Check sheet for the modelled part. Datum: model origin and axes. Units: mm. A direction names the side the tool comes from. Round coordinates to 2 decimals unless told otherwise and drop trailing zeros. Write each loop counter-clockwise with the first axis right and the second up, starting at its lowest first coordinate (ties: lowest second). Pieces come first, ordered by that corner, then holes.
Item 1: Section check C-C, the plane x = 7.75. Record the cut outline in (y, z).
Item 2: Material ranges on line 1 along X through (y, z) = (3.25, 0.8); line 2 along Y through (x, z) = (6.5, 0.45); line 3 along X through (y, z) = (3, 0.8), recorded low to high.
Item 3: Set-up check for faces 1 (the flat face through (0, 7.5, 0.5)), 2 (the cylindrical face through (4.977, -0.483, 0.493)), 3 (the cylindrical face through (-4.413, 2.351, 0.493)), 4 (the flat face through (-1.47, -7.39, 0.49)): record each of +Z, -Z, +X, -X, +Y, -Y from which the full face is reachable in a straight line by a thin tool's end or side.
Item 4: Section check B-B, the plane y = 6. Record the cut outline in (x, z), plus the area to 3 significant figures.
Item 5: Release check for a two-part mould opening along Y. For faces 5 (the flat face through (7.702, -6.303, 0.493)), 6 (the flat face through (-1, 9.9, 0.5)), 7 (the flat face through (-7, 2.9, 0.5)) record: pulls with the +Y half, pulls with the -Y half, needs draft (parallel to the pull), parting line crosses it, or undercut.
Item 6: Section check A-A, the plane x = -3.25. Record the cut outline in (y, z).
Item 7: Depth check by flat-ended pin: pin 1 (2 mm diameter, centred on x = 4.5, y = -4.5, fed in from -Z). Enter the tip coordinate at first touch or a pass-through.
Autodesk Inventor part; units mm, degrees
ref_plane "YZ Plane" through (0, 0, 0) normal (1, 0, 0) x (0, 1, 0)
ref_plane "XZ Plane" through (0, 0, 0) normal (0, 1, 0) x (-1, 0, 0)
ref_plane "XY Plane" through (0, 0, 0) normal (0, 0, 1) x (1, 0, 0)
sketch "Sketch1" plane through (0, 0, 0) normal (0, 0, 1) x (1, 0, 0)
  circle A0 centre (0, 0) radius 1
  circle A1 centre (0, 0) radius 5
  line L0 (1.9509, 9.8079) -> (3.8268, 9.2388)
  line L1 (5.5557, 8.3147) -> (7.0711, 7.0711)
  line L2 (8.3147, 5.5557) -> (9.2388, 3.8268)
  line L3 (9.8079, 1.9509) -> (10, 0)
  line L4 (9.8079, -1.9509) -> (9.2388, -3.8268)
  line L5 (8.3147, -5.5557) -> (7.0711, -7.0711)
  line L6 (5.5557, -8.3147) -> (3.8268, -9.2388)
  line L7 (1.9509, -9.8079) -> (0, -10)
  line L8 (-1.9509, -9.8079) -> (-3.8268, -9.2388)
  line L9 (-5.5557, -8.3147) -> (-7.0711, -7.0711)
  line L10 (-8.3147, -5.5557) -> (-9.2388, -3.8268)
  line L11 (-9.8079, -1.9509) -> (-10, 0)
  line L12 (-9.8079, 1.9509) -> (-9.2388, 3.8268)
  line L13 (-8.3147, 5.5557) -> (-7.0711, 7.0711)
  line L14 (-5.5557, 8.3147) -> (-3.8268, 9.2388)
  line L15 (-1.9509, 9.8079) -> (0, 10)
  line L16 (-3.8268, 9.2388) -> (-1.9134, 4.6194)
  line L17 (-5.5557, 8.3147) -> (-2.7779, 4.1573)
  line L18 (-9.2388, -3.8268) -> (-4.6194, -1.9134)
  line L19 (-8.3147, -5.5557) -> (-4.1573, -2.7779)
  line L20 (-7.0711, -7.0711) -> (-3.5355, -3.5355)
  line L21 (-5.5557, -8.3147) -> (-2.7779, -4.1573)
  line L22 (-1.9509, -9.8079) -> (-0.9755, -4.9039)
  line L23 (-3.8268, -9.2388) -> (-1.9134, -4.6194)
  line L24 (0, -5) -> (0, -10)
  line L25 (0.9755, -4.9039) -> (1.9509, -9.8079)
  line L26 (-0.3827, 0.9239) -> (0.3827, -0.9239)
  line L27 (1.9134, -4.6194) -> (3.8268, -9.2388)
  line L28 (-0.5556, 0.8315) -> (0.5556, -0.8315)
  line L29 (2.7779, -4.1573) -> (5.5557, -8.3147)
  line L30 (3.5355, -3.5355) -> (7.0711, -7.0711)
  line L31 (4.1573, -2.7779) -> (8.3147, -5.5557)
  line L32 (4.6194, -1.9134) -> (9.2388, -3.8268)
  line L33 (4.9039, -0.9755) -> (9.8079, -1.9509)
  line L34 (5, 0) -> (10, 0)
  line L35 (4.9039, 0.9755) -> (9.8079, 1.9509)
  line L36 (-0.9239, -0.3827) -> (0.9239, 0.3827)
  line L37 (4.6194, 1.9134) -> (9.2388, 3.8268)
  line L38 (-0.8315, -0.5556) -> (0.8315, 0.5556)
  line L39 (4.1573, 2.7779) -> (8.3147, 5.5557)
  line L40 (-0.7071, -0.7071) -> (0.7071, 0.7071)
  line L41 (3.5355, 3.5355) -> (7.0711, 7.0711)
  line L42 (-0.5556, -0.8315) -> (0.5556, 0.8315)
  line L43 (2.7779, 4.1573) -> (5.5557, 8.3147)
  line L44 (-0.3827, -0.9239) -> (0.3827, 0.9239)
  line L45 (1.9134, 4.6194) -> (3.8268, 9.2388)
  line L46 (-0.1951, -0.9808) -> (0.1951, 0.9808)
  line L47 (0.9755, 4.9039) -> (1.9509, 9.8079)
  line L48 (0, 10) -> (0, 5)
  line L49 (0, 1) -> (0, -1)
  line L50 (-1.9509, 9.8079) -> (-0.9755, 4.9039)
  line L51 (-0.1951, 0.9808) -> (0.1951, -0.9808)
  line L52 (-7.0711, 7.0711) -> (-3.5355, 3.5355)
  line L53 (-0.7071, 0.7071) -> (0.7071, -0.7071)
  line L54 (-8.3147, 5.5557) -> (-4.1573, 2.7779)
  line L55 (-0.8315, 0.5556) -> (0.8315, -0.5556)
  line L56 (-9.2388, 3.8268) -> (-4.6194, 1.9134)
  line L57 (-0.9239, 0.3827) -> (0.9239, -0.3827)
  line L58 (-0.9808, 0.1951) -> (0.9808, -0.1951)
  line L59 (-10, 0) -> (-5, 0)
  line L60 (-1, 0) -> (1, 0)
  line L61 (-9.8079, -1.9509) -> (-4.9039, -0.9755)
  line L62 (-0.9808, -0.1951) -> (0.9808, 0.1951)
  line L63 (-9.8079, 1.9509) -> (-4.9039, 0.9755)
  line L64 (-0.9808, 0.1951) -> (0, 0)
  dimension "d1" = 2
extrude "Extrusion2" add sketch "Sketch1" along normal blind 1
properties part number "encoder"
Values found:
1. outline: (-6.24, 0) - (-5.18, 0) - (-5.18, 1) - (-6.24, 1) - close; (-3.21, 0) - (-1.54, 0) - (-1.54, 1) - (-3.21, 1) - close; (0, 0) - (1.54, 0) - (1.54, 1) - (0, 1) - close; (3.21, 0) - (5.18, 0) - (5.18, 1) - (3.21, 1) - close
2. line 1: x = -9.41 to -7.85, -4.86 to 3.8, 4.86 to 7.85
2. line 2: y = -6.5 to -4.34, -2.69 to -1.29, 0 to 1.29, 2.69 to 4.34, 6.5 to 7.54
2. line 3: x = -9.49 to -7.24, -4.49 to 4, 4.49 to 7.24
3. face 1: +Z, -Z, +Y
3. face 2: +Z, -Z, +X
3. face 3: +Z, -Z
3. face 4: +Z, -Z, -Y
4. outline: (-7.95, 0) - (-6, 0) - (-6, 1) - (-7.95, 1) - close; (-4.01, 0) - (-2.49, 0) - (-2.49, 1) - (-4.01, 1) - close; (-1.19, 0) - (0, 0) - (0, 1) - (-1.19, 1) - close; (1.19, 0) - (2.49, 0) - (2.49, 1) - (1.19, 1) - close; (4.01, 0) - (6, 0) - (6, 1) - (4.01, 1) - close
4. area: 7.95 mm2
5. face 5: pulls with the -Y half
5. face 6: pulls with the +Y half
5. face 7: undercut
6. outline: (-9.41, 0) - (-7.85, 0) - (-7.85, 1) - (-9.41, 1) - close; (-4.86, 0) - (3.8, 0) - (3.8, 1) - (-4.86, 1) - close; (4.86, 0) - (7.85, 0) - (7.85, 1) - (4.86, 1) - close
7. pin 1: stops at z = 0
